Part print with two shaded views. Sizes in mm from the minimum x, y, z corner. Round coordinates to 2 decimals unless told otherwise and drop trailing zeros. Write each loop counter-clockwise with the first axis right and the second up, starting at its lowest first coordinate (ties: lowest second). Pieces come first, ordered by that corner, then holes. Notation, with made-up numbers: (17, -22.5) - (41, -22.5) arc R23 ccw to (41, -8.5) - close; hole circle Ø4 at (7, -5.5). An arc over 180 degrees is marked (long way). Use one line per item in the form item = value. Start each with the question number.
Item 1: Drill centre lines: L1, parallel to X at y = 1.3, z = 8; L2, parallel to X at y = 2.8, z = 66.5; L3, parallel to Z at x = 4, y = 0.7. Where is each one in solid material? Low to high.
Item 2: Band-saw the part on B-B, the plane y = 3.55. List the corners of the cut face in (x, z), and give its area (3 significant figures).
Item 3: Pin check, flat tip, straight feed: pin 1 (2.5 mm diameter, centred on y = 1.5, z = 9.5, fed in from -X). Stop position of the tip, or through.
Item 4: Band-saw the part on D-D, the plane z = 24. List the corners of the cut face in (x, y), and give its area (3 significant figures).
Item 5: Band-saw the part on A-A, the plane z = 16. List the corners of the cut face in (x, y).
Item 6: Band-saw the part on C-C, the plane x = 65.84. List the corners of the cut face in (y, z), and give its area (3 significant figures).
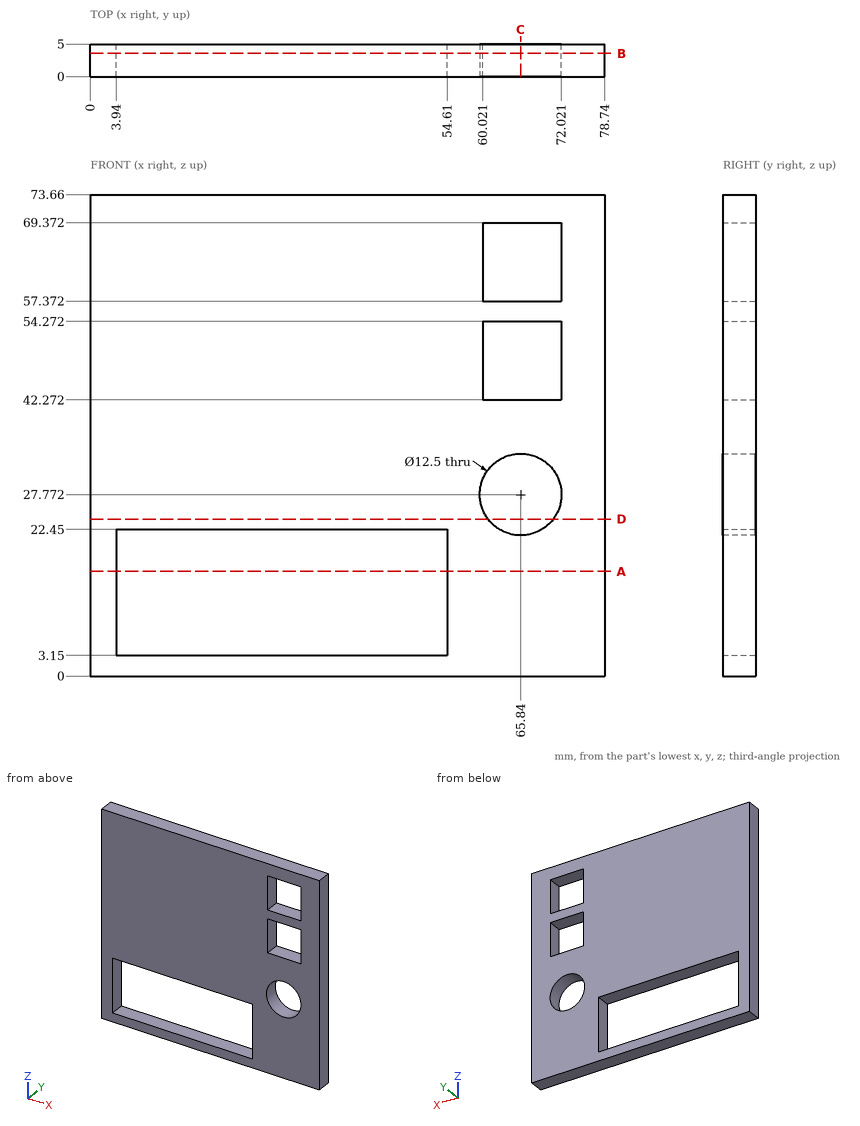
Determined:
q1.L1 = 0 to 3.94, 54.61 to 78.74
q1.L2 = 0 to 60.02, 72.02 to 78.74
q1.L3 = 0 to 3.15, 22.45 to 73.66
q2.outline = (0, 0) - (78.74, 0) - (78.74, 73.66) - (0, 73.66) - close; hole (3.94, 3.15) - (54.61, 3.15) - (54.61, 22.45) - (3.94, 22.45) - close; hole circle Ø12.5 at (65.84, 27.77); hole (60.02, 42.27) - (72.02, 42.27) - (72.02, 54.27) - (60.02, 54.27) - close; hole (60.02, 57.37) - (72.02, 57.37) - (72.02, 69.37) - (60.02, 69.37) - close
q2.area = 4,410 mm²
q3.pin_1 = 0
q4.outline = (0, 0) - (60.86, 0) - (60.86, 5) - (0, 5) - close; (70.82, 0) - (78.74, 0) - (78.74, 5) - (70.82, 5) - close
q4.area = 344 mm²
q5.outline = (0, 0) - (3.94, 0) - (3.94, 5) - (0, 5) - close; (54.61, 0) - (78.74, 0) - (78.74, 5) - (54.61, 5) - close
q6.outline = (0, 0) - (5, 0) - (5, 21.52) - (0, 21.52) - close; (0, 34.02) - (5, 34.02) - (5, 42.27) - (0, 42.27) - close; (0, 54.27) - (5, 54.27) - (5, 57.37) - (0, 57.37) - close; (0, 69.37) - (5, 69.37) - (5, 73.66) - (0, 73.66) - close
q6.area = 186 mm²
